Design review of the part built by this model. Coordinates are the model's own, in mm. Round coordinates to 2 decimals unless told otherwise and drop trailing zeros. Write each loop counter-clockwise with the first axis right and the second up, starting at its lowest first coordinate (ties: lowest second). Pieces come first, ordered by that corner, then holes.
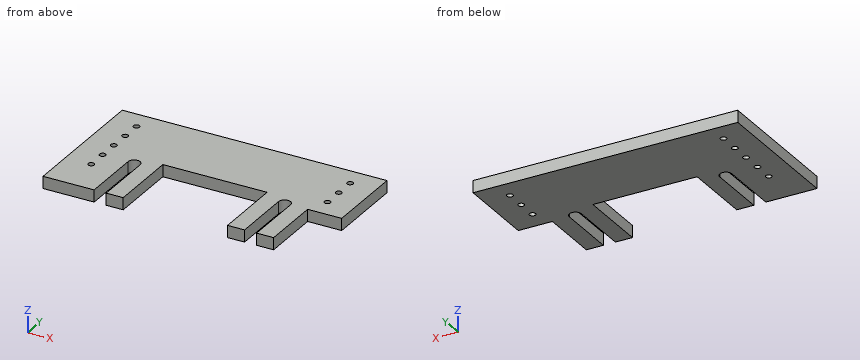
from build123d import *

# Parameters (mm, degrees)
ESBO_O1_R                = 1.5
RESSALTO_EXTRUS_O1_DEPTH = 6


with BuildPart() as part:
    # Esboço1 → Ressalto-extrusão1 (new body)
    with BuildSketch(Plane.XY):
        with BuildLine():
            Line((-66, -35), (-40.5, -35))
            Line((-40.5, -35), (-40.5, -5))
            ThreePointArc((-40.5, -5), (-37.5, -2), (-34.5, -5))
            Line((-34.5, -5), (-34.5, -35))
            Line((-34.5, -35), (-26, -35))
            Line((-26, -35), (-26, 0))
            Line((-26, 0), (26, 0))
            Line((26, 0), (26, -35))
            Line((26, -35), (34.5, -35))
            Line((34.5, -35), (34.5, -5))
            ThreePointArc((34.5, -5), (37.5, -2), (40.5, -5))
            Line((40.5, -5), (40.5, -35))
            Line((40.5, -35), (49, -35))
            Line((49, -35), (49, -5))
            Line((49, -5), (66, -5))
            Line((66, -5), (66, 35))
            Line((66, 35), (-66, 35))
            Line((-66, 35), (-66, -35))
        make_face()
        with Locations((-53.25, -5)):
            Circle(ESBO_O1_R, mode=Mode.SUBTRACT)
        with Locations((-53.25, -15)):
            Circle(ESBO_O1_R, mode=Mode.SUBTRACT)
        with Locations((-53.25, 15)):
            Circle(ESBO_O1_R, mode=Mode.SUBTRACT)
        with Locations((-53.25, 25)):
            Circle(ESBO_O1_R, mode=Mode.SUBTRACT)
        with Locations((-53.25, 5)):
            Circle(ESBO_O1_R, mode=Mode.SUBTRACT)
        with Locations((53.25, 5)):
            Circle(ESBO_O1_R, mode=Mode.SUBTRACT)
        with Locations((53.25, 25)):
            Circle(ESBO_O1_R, mode=Mode.SUBTRACT)
        with Locations((53.25, 15)):
            Circle(ESBO_O1_R, mode=Mode.SUBTRACT)
    extrude(amount=RESSALTO_EXTRUS_O1_DEPTH)


solid = part.part
1) For P1, Ø3, axis at x = 60.5, z = 3, coming from the -Y side; P2, Ø4, axis at x = 53.25, y = 25, coming from the -Z side; P3, Ø1.8, axis at y = -14, z = 2.5, coming from the +X side, all flat-tipped, find the tip position at first contact; note any pin that passes through.
2) Add section C-C on y = -15. State the section outline as (x, z) points, and give its area (3 significant figures).
3) For line 1 along Y through (x, z) = (53.5, 5.2); line 2 along Y through (x, z) = (-53.25, 4.15); line 3 along X through (y, z) = (-12, 4), list the stretches that pass through material, from the lowest coordinate up.
4) Add section D-D on z = 4.3. Count the separate pieces of the cut face and the enclosed holes in it, and give its area (3 significant figures).
5) Add section B-B on x = -53.25. State the section outline as (y, z) points, and give its area (3 significant figures).
6) Add section A-A on y = 5. State the section outline as (x, z) points, and give its area (3 significant figures).
Computed:
1. P1: stops at y = -5
1. P2: stops at z = 0
1. P3: stops at x = 49
2. outline: (-66, 0) - (-54.75, 0) - (-54.75, 6) - (-66, 6) - close; (-51.75, 0) - (-40.5, 0) - (-40.5, 6) - (-51.75, 6) - close; (-34.5, 0) - (-26, 0) - (-26, 6) - (-34.5, 6) - close; (26, 0) - (34.5, 0) - (34.5, 6) - (26, 6) - close; (40.5, 0) - (49, 0) - (49, 6) - (40.5, 6) - close
2. area: 288 mm2
3. line 1: y = -5 to 3.52, 6.48 to 13.52, 16.48 to 23.52, 26.48 to 35
3. line 2: y = -35 to -16.5, -13.5 to -6.5, -3.5 to 3.5, 6.5 to 13.5, 16.5 to 23.5, 26.5 to 35
3. line 3: x = -66 to -40.5, -34.5 to -26, 26 to 34.5, 40.5 to 49
4. separate pieces: 1
4. enclosed holes: 8
4. area: 6,470 mm2
5. outline: (-35, 0) - (-16.5, 0) - (-16.5, 6) - (-35, 6) - close; (-13.5, 0) - (-6.5, 0) - (-6.5, 6) - (-13.5, 6) - close; (-3.5, 0) - (3.5, 0) - (3.5, 6) - (-3.5, 6) - close; (6.5, 0) - (13.5, 0) - (13.5, 6) - (6.5, 6) - close; (16.5, 0) - (23.5, 0) - (23.5, 6) - (16.5, 6) - close; (26.5, 0) - (35, 0) - (35, 6) - (26.5, 6) - close
5. area: 330 mm2
6. outline: (-66, 0) - (-54.75, 0) - (-54.75, 6) - (-66, 6) - close; (-51.75, 0) - (51.75, 0) - (51.75, 6) - (-51.75, 6) - close; (54.75, 0) - (66, 0) - (66, 6) - (54.75, 6) - close
6. area: 756 mm2
